Part model, mm, in its own coordinate system. Round coordinates to 2 decimals unless told otherwise and drop trailing zeros. Loops run counter-clockwise (first coordinate to the right, second up) from the corner with the lowest first, then second, coordinate; pieces in that order, holes last.
1) Band-saw the part on C-C, the plane x = -117.8. State how many separate pieces and enclosed holes the cut face has, then the cut area to 3 significant figures.
2) Drop flat-ended pins along their axis: P1, Ø0.7, axis at x = -118, y = 1.5, coming from the -Z side; P2, Ø1.5, axis at x = -117, y = 43, coming from the +Z side; P3, Ø0.6, axis at x = -117.5, z = 70.5, coming from the -Y side; P4, Ø1.5, axis at x = -117, z = 136, coming from the +Y side (3 decimals). Give the stop position or say it passes through.
3) Band-saw the part on B-B, the plane y = 74. Write the cut outline in (x, z).
4) Probe line 1 (Y direction, x = -116.6, z = 98); line 2 (Z direction, x = -116.8, y = 9); line 3 (Y direction, x = -116.4, z = -36). List the from-to ranges inside material, lowest first.
5) Band-saw the part on A-A, the plane z = -51. Write the cut outline in (x, y).
from build123d import *

# Parameters (mm, degrees)
BOSS_EXTRUDE1_DEPTH = 2.9


with BuildPart() as part:
    # Sketch1 → Boss-Extrude1 (new body)
    with BuildSketch(Plane(origin=(-118.9, 0, 0), x_dir=(0, 0, -1), z_dir=(1, 0, 0))):
        Polygon((135, 2.9), (110, 2.9), (110, 0.5), (109.5, 0), (80.5, 0), (80, 0.5), (80, 2.9), (15, 2.9), (15, 0.5), (14.5, 0), (-14.5, 0), (-15, 0.5), (-15, 2.9), (-60, 2.9), (-60, 0.5), (-60.5, 0), (-89.5, 0), (-90, 0.5), (-90, 2.9), (-135, 2.9), (-135, 18.725), (-137.9, 18.725), (-137.9, 34.475), (-135, 34.475), (-135, 50.325), (-137.9, 50.325), (-137.9, 66.075), (-135, 66.075), (-135, 81.9), (-90, 81.9), (-90, 84.3), (-89.5, 84.8), (-60.5, 84.8), (-60, 84.3), (-60, 81.9), (80, 81.9), (80, 84.3), (80.5, 84.8), (109.5, 84.8), (110, 84.3), (110, 81.9), (135, 81.9), (135, 66.075), (137.9, 66.075), (137.9, 50.325), (135, 50.325), (135, 34.475), (137.9, 34.475), (137.9, 18.725), (135, 18.725), align=None)
        with BuildLine():
            Line((-114.5, 30), (-116.5, 30))
            ThreePointArc((-116.5, 30), (-116.853553391, 30.146446609), (-117, 30.5))
            Line((-117, 30.5), (-117, 54.5))
            ThreePointArc((-117, 54.5), (-116.853553391, 54.853553391), (-116.5, 55))
            Line((-116.5, 55), (-114.5, 55))
            ThreePointArc((-114.5, 55), (-114.146446609, 54.853553391), (-114, 54.5))
            Line((-114, 54.5), (-114, 30.5))
            ThreePointArc((-114, 30.5), (-114.146446609, 30.146446609), (-114.5, 30))
        make_face(mode=Mode.SUBTRACT)
        with BuildLine():
            Line((-105.5, 30), (-107.5, 30))
            ThreePointArc((-107.5, 30), (-107.853553391, 30.146446609), (-108, 30.5))
            Line((-108, 30.5), (-108, 54.5))
            ThreePointArc((-108, 54.5), (-107.853553391, 54.853553391), (-107.5, 55))
            Line((-107.5, 55), (-105.5, 55))
            ThreePointArc((-105.5, 55), (-105.146446609, 54.853553391), (-105, 54.5))
            Line((-105, 54.5), (-105, 30.5))
            ThreePointArc((-105, 30.5), (-105.146446609, 30.146446609), (-105.5, 30))
        make_face(mode=Mode.SUBTRACT)
        with BuildLine():
            Line((-96.5, 30), (-98.5, 30))
            ThreePointArc((-98.5, 30), (-98.853553391, 30.146446609), (-99, 30.5))
            Line((-99, 30.5), (-99, 54.5))
            ThreePointArc((-99, 54.5), (-98.853553391, 54.853553391), (-98.5, 55))
            Line((-98.5, 55), (-96.5, 55))
            ThreePointArc((-96.5, 55), (-96.146446609, 54.853553391), (-96, 54.5))
            Line((-96, 54.5), (-96, 30.5))
            ThreePointArc((-96, 30.5), (-96.146446609, 30.146446609), (-96.5, 30))
        make_face(mode=Mode.SUBTRACT)
        with BuildLine():
            Line((-87.5, 30), (-89.5, 30))
            ThreePointArc((-89.5, 30), (-89.853553391, 30.146446609), (-90, 30.5))
            Line((-90, 30.5), (-90, 54.5))
            ThreePointArc((-90, 54.5), (-89.853553391, 54.853553391), (-89.5, 55))
            Line((-89.5, 55), (-87.5, 55))
            ThreePointArc((-87.5, 55), (-87.146446609, 54.853553391), (-87, 54.5))
            Line((-87, 54.5), (-87, 30.5))
            ThreePointArc((-87, 30.5), (-87.146446609, 30.146446609), (-87.5, 30))
        make_face(mode=Mode.SUBTRACT)
        with BuildLine():
            Line((-78.5, 30), (-80.5, 30))
            ThreePointArc((-80.5, 30), (-80.853553391, 30.146446609), (-81, 30.5))
            Line((-81, 30.5), (-81, 54.5))
            ThreePointArc((-81, 54.5), (-80.853553391, 54.853553391), (-80.5, 55))
            Line((-80.5, 55), (-78.5, 55))
            ThreePointArc((-78.5, 55), (-78.146446609, 54.853553391), (-78, 54.5))
            Line((-78, 54.5), (-78, 30.5))
            ThreePointArc((-78, 30.5), (-78.146446609, 30.146446609), (-78.5, 30))
        make_face(mode=Mode.SUBTRACT)
        with BuildLine():
            Line((-69.5, 30), (-71.5, 30))
            ThreePointArc((-71.5, 30), (-71.853553391, 30.146446609), (-72, 30.5))
            Line((-72, 30.5), (-72, 54.5))
            ThreePointArc((-72, 54.5), (-71.853553391, 54.853553391), (-71.5, 55))
            Line((-71.5, 55), (-69.5, 55))
            ThreePointArc((-69.5, 55), (-69.146446609, 54.853553391), (-69, 54.5))
            Line((-69, 54.5), (-69, 30.5))
            ThreePointArc((-69, 30.5), (-69.146446609, 30.146446609), (-69.5, 30))
        make_face(mode=Mode.SUBTRACT)
        with BuildLine():
            Line((-60.5, 30), (-62.5, 30))
            ThreePointArc((-62.5, 30), (-62.853553391, 30.146446609), (-63, 30.5))
            Line((-63, 30.5), (-63, 54.5))
            ThreePointArc((-63, 54.5), (-62.853553391, 54.853553391), (-62.5, 55))
            Line((-62.5, 55), (-60.5, 55))
            ThreePointArc((-60.5, 55), (-60.146446609, 54.853553391), (-60, 54.5))
            Line((-60, 54.5), (-60, 30.5))
            ThreePointArc((-60, 30.5), (-60.146446609, 30.146446609), (-60.5, 30))
        make_face(mode=Mode.SUBTRACT)
    extrude(amount=BOSS_EXTRUDE1_DEPTH)


solid = part.part
Reported:
1. separate pieces: 1
1. enclosed holes: 7
1. area: 21,400 mm2
2. P1: stops at z = -110
2. P2: stops at z = 135
2. P3: stops at y = 0
2. P4: stops at y = 66.075
3. outline: (-118.9, -135) - (-116, -135) - (-116, 135) - (-118.9, 135) - close
4. line 1: y = 2.9 to 30, 55 to 81.9
4. line 2: z = -135 to 135
4. line 3: y = 2.9 to 81.9
5. outline: (-118.9, 2.9) - (-116, 2.9) - (-116, 81.9) - (-118.9, 81.9) - close
